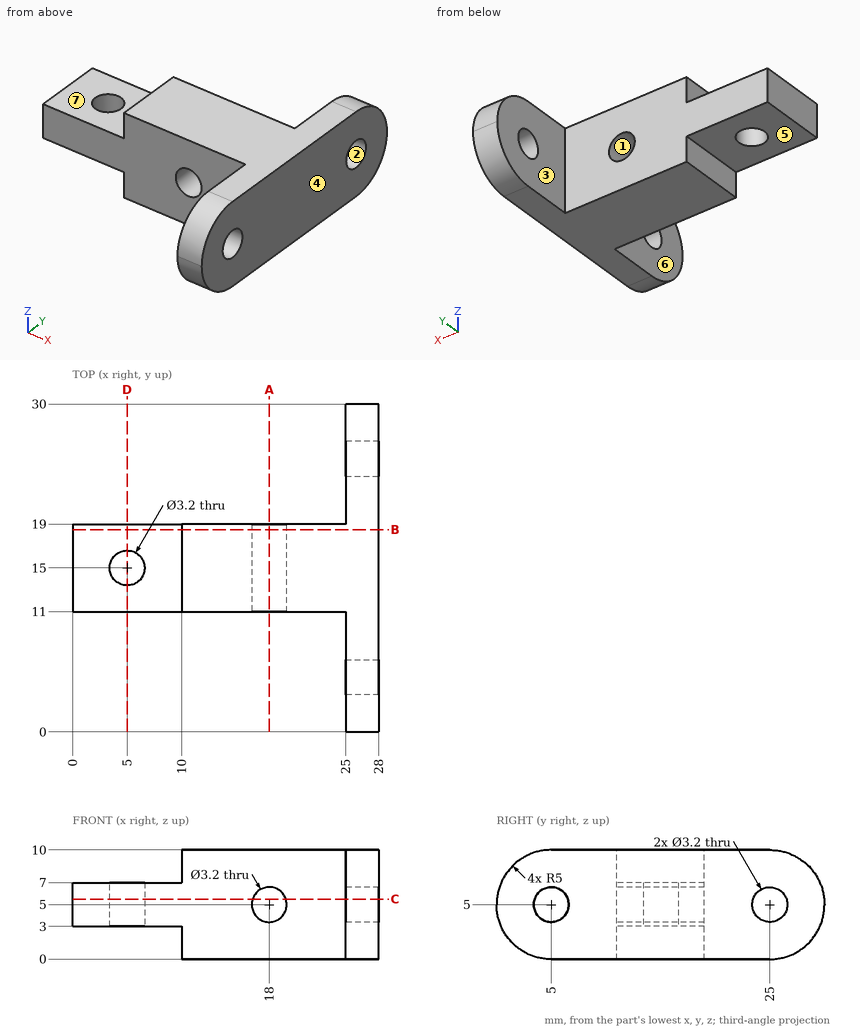
Design review of the part shown in the three views and the two pictorial views. Dimensions are in mm from the part's minimum x, y and z. A direction names the side the tool comes from. Give positions to 0.01 mm unless a question says otherwise; leave off trailing zeros. Write each loop counter-clockwise with the first axis right and the second up, starting at its lowest first coordinate (ties: lowest second). Pieces come first, ordered by that corner, then holes.
(1) Wall thickness on line 1 along Y through (x, z) = (5, 5.75); line 2 along Y through (x, z) = (14, 6.5); line 3 along X through (y, z) = (12.25, 8.25): over which ranges is each line inside the solid? List them lowest first.
Checked values:
line 1: y = 11 to 13.4, 16.6 to 19
line 2: y = 11 to 19
line 3: x = 10 to 28
(2) Clearance check with flat-ended pins moving along their axes: pin 1 Ø1 at (y, z) = (22.5, 6.5) entering from -X; pin 2 Ø2.5 at (x, y) = (2.5, 15.5) entering from -Z; pin 3 Ø0.9 at (y, z) = (14.5, 8) entering from -X. State where each tip first meets the part, or that it passes through.
Checked values:
pin 1: stops at x = 25
pin 2: stops at z = 3
pin 3: stops at x = 10
(3) Tool access review of the marked faces 5, 6 and 7: name each direction out of +Z, -Z, +X, -X, +Y, -Y from which nothing blocks a thin tool from reaching the whole face with its end or side.
Checked values:
face 5: -Z, -X, +Y, -Y
face 6: +Z, -Z, -X, -Y
face 7: +Z, -X, +Y, -Y
(4) Add section C-C (z = 5.5). Give the boundary of the cut face in (x, y) (3 decimals).
Checked values:
outline: (0, 11) - (16.48, 11) - (16.48, 19) - (0, 19) - close; (19.52, 11) - (25, 11) - (25, 6.52) - (28, 6.52) - (28, 23.48) - (25, 23.48) - (25, 19) - (19.52, 19) - close; (25, 0.025) - (28, 0.025) - (28, 3.48) - (25, 3.48) - close; (25, 26.52) - (28, 26.52) - (28, 29.975) - (25, 29.975) - close; hole circle Ø3.2 at (5, 15)
(5) Add section D-D (x = 5). Give the boundary of the cut face in (y, z), and give its area (3 significant figures).
Checked values:
outline: (11, 3) - (13.4, 3) - (13.4, 7) - (11, 7) - close; (16.6, 3) - (19, 3) - (19, 7) - (16.6, 7) - close
area: 19.2 mm2
(6) Mouldability with a two-part tool opening along X and no side actions: class the marked faces 1, 2, 3 and 4 as +X half, -X half, draft (parallel to the pull), parting line (faces both ways), or undercut.
Checked values:
face 1: undercut
face 2: draft
face 3: -X half
face 4: +X half
(7) Add section B-B (y = 18.5). Give the boundary of the cut face in (x, z), and give its area (3 significant figures).
Checked values:
outline: (0, 3) - (10, 3) - (10, 0) - (28, 0) - (28, 10) - (10, 10) - (10, 7) - (0, 7) - close; hole circle Ø3.2 at (18, 5)
area: 212 mm2
(8) Add section A-A (x = 18). Give the boundary of the cut face in (y, z), and give its area (3 significant figures).
Checked values:
outline: (11, 0) - (19, 0) - (19, 3.4) - (11, 3.4) - close; (11, 6.6) - (19, 6.6) - (19, 10) - (11, 10) - close
area: 54.4 mm2
